Job drawing, mm, ordinate dimensions from the low corner. One solid piece. A direction names the side the tool comes from. Round coordinates to 2 decimals unless told otherwise and drop trailing zeros. Loops run counter-clockwise (first coordinate to the right, second up) from the corner with the lowest first, then second, coordinate; pieces in that order, holes last. Notation, with made-up numbers: M 61.25,-16.75 L 117.25,-16.75 A31 cw 117.25,22.25 Z; hole C 30.25,88.25 d10. An arc over 180 degrees is marked long. Put each result on its own line as item: value. Start each with the question number.
1) Pull direction Y, two halves, no side cores. Call the marked faces 4, 5 and 6: +Y half, -Y half, draft (parallel to the pull), parting line (faces both ways), or undercut.
2) Which spindle directions (+Z, -Z, +X, -X, +Y, -Y) get a long thin tool onto all of the face, cutting with end or side? Do the marked faces 1, 2 and 3. Say none if no direction does.
3) Slice it at C-C on y = 10.5. Give the cut face in (x, z).
4) Slice it at A-A on z = 24. Give the cut face in (x, y), then the cut area to 3 significant figures.
5) Drop flat-ended pins along their axis: pin 1 Ø0.5 at (x, y) = (5, 12) entering from -Z; pin 2 Ø3 at (x, y) = (6.35, 6.35) entering from -Z; pin 3 Ø2 at (x, z) = (3.5, 27) entering from +Y (1 decimal); pin 4 Ø6.5 at (x, z) = (6, 16) entering from +Y. Give the stop position or say it passes through.
6) Probe line 1 along Y through (x, z) = (6.35, 5.5); line 2 along Z through (x, y) = (9.5, 7.25); line 3 along Y through (x, z) = (5, 9) (1 decimal). List the from-to ranges inside material, lowest first.
7) Slice it at D-D on x = 1.25. Give the cut face in (y, z).
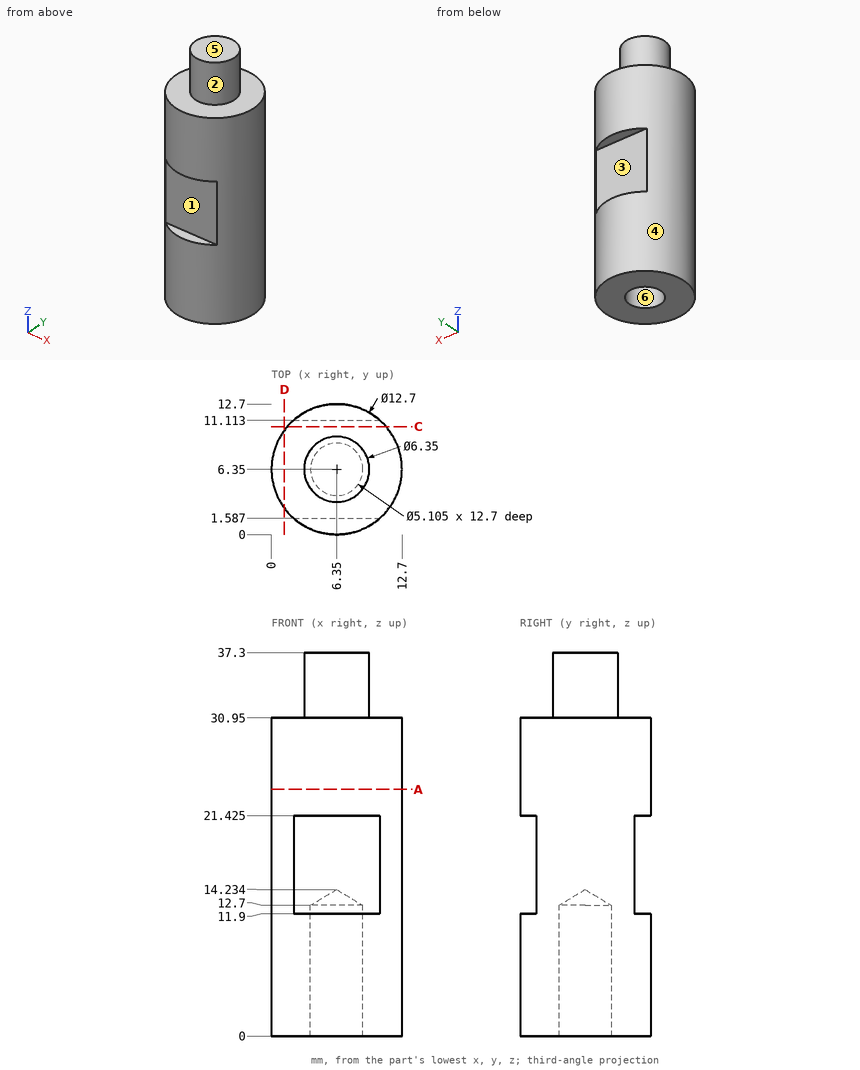
Recorded:
1. face 4: parting line
1. face 5: draft
1. face 6: undercut
2. face 1: +X, -X, -Y
2. face 2: +Z
2. face 3: +X, -X, +Y
3. outline: M 1.54,0 L 11.16,0 L 11.16,30.95 L 1.54,30.95 Z
4. outline: C 6.35,6.35 d12.7
4. area: 127 mm2
5. pin 1: stops at z = 0
5. pin 2: stops at z = 13.33
5. pin 3: stops at y = 12.4
5. pin 4: stops at y = 11.11
6. line 1: y = 0 to 3.8, 8.9 to 12.7
6. line 2: z = 0 to 30.95
6. line 3: y = 0.1 to 4.2, 8.5 to 12.6
7. outline: M 2.57,0 L 10.13,0 L 10.13,30.95 L 2.57,30.95 Z
